CAD build for the part. Positions are in the model's coordinates, mm. A direction names the side the tool comes from. Give positions to 0.01 mm unless a question says otherwise; leave off trailing zeros. Write each loop counter-clockwise with the first axis right and the second up, starting at its lowest first coordinate (ties: lowest second). Pieces come first, ordered by that corner, then holes. Notation, with made-up numbers: (-10, -33.75) -> (-5, -33.75) arc R25 cw to (-5, -20.75) -> close; hole circle Ø9 at (-16, -36.5). An arc over 180 degrees is marked (long way). Answer as a JSON object with one key per item and string values.
```python
from build123d import *

# Parameters (mm, degrees)
ESQUISSE1_R        = 4.4
BOSS_EXTRU_1_DEPTH = 3
ESQUISSE2_R        = 7
BOSS_EXTRU_2_DEPTH = 2
ESQUISSE3_R        = 6.35
BOSS_EXTRU_3_DEPTH = 10
ESQUISSE4_R        = 4
BOSS_EXTRU_4_DEPTH = 7
ESQUISSE5_W        = 0.4
ESQUISSE5_H        = 2
BOSS_EXTRU_5_DEPTH = 5.8


with BuildPart() as part:
    # Esquisse1 → Boss.-Extru.1 (new body)
    with BuildSketch(Plane.XY):
        Circle(ESQUISSE1_R)
    extrude(amount=BOSS_EXTRU_1_DEPTH)

    # Esquisse2 → Boss.-Extru.2 (add)
    with BuildSketch(Plane.XY.offset(3)):
        Circle(ESQUISSE2_R)
    extrude(amount=BOSS_EXTRU_2_DEPTH)

    # Esquisse3 → Boss.-Extru.3 (add)
    with BuildSketch(Plane.XY.offset(5)):
        Circle(ESQUISSE3_R)
    extrude(amount=BOSS_EXTRU_3_DEPTH)

    # Esquisse4 → Boss.-Extru.4 (add)
    with BuildSketch(Plane.XY.offset(15)):
        Circle(ESQUISSE4_R)
    extrude(amount=BOSS_EXTRU_4_DEPTH)

    # Esquisse5 → Boss.-Extru.5 (add)
    with BuildSketch(Plane.XY.offset(22)):
        with Locations((-2.2, 0)):
            Rectangle(ESQUISSE5_W, ESQUISSE5_H)
        with Locations((2.2, 0)):
            Rectangle(ESQUISSE5_W, ESQUISSE5_H)
    extrude(amount=BOSS_EXTRU_5_DEPTH)


solid = part.part
```
1) 3-axis set-ups, long thin cutter, end or side, ignore diameter. For faces 1 (the cylindrical face through (-1.38, -6.2, 9.93)), 2 (the flat face through (0, -5, 3)), 3 (the flat face through (-2, 0, 25)): which of +Z, -Z, +X, -X, +Y, -Y reach the whole face in a straight line?
Model answer:
{"face 1": "+Z", "face 2": "-Z", "face 3": "+Z, +Y, -Y"}
2) Slice it at B-B (y = 0). List the corners of the cut face in (x, z).
Model answer:
{"outline": "(-7, 3) -> (-4.4, 3) -> (-4.4, 0) -> (4.4, 0) -> (4.4, 3) -> (7, 3) -> (7, 5) -> (6.35, 5) -> (6.35, 15) -> (4, 15) -> (4, 22) -> (2.4, 22) -> (2.4, 27.8) -> (2, 27.8) -> (2, 22) -> (-2, 22) -> (-2, 27.8) -> (-2.4, 27.8) -> (-2.4, 22) -> (-4, 22) -> (-4, 15) -> (-6.35, 15) -> (-6.35, 5) -> (-7, 5) -> close"}
3) Pin check, flat tips, straight feed: pin 1 (3 mm diameter, centred on x = -5.5, z = 12.5, fed in from -Y); pin 2 (5 mm diameter, centred on x = -3.5, z = 19, fed in from -Y); pin 3 (1.6 mm diameter, centred on y = -0.5, z = 24.5, fed in from +X). Stop position of each tip, or through.
Model answer:
{"pin 1": "stops at y = -4.93", "pin 2": "stops at y = -3.87", "pin 3": "stops at x = 2.4"}
4) Slice it at C-C (x = 0). List the corners of the cut face in (y, z), then the cut area to 3 significant figures.
Model answer:
{"outline": "(-7, 3) -> (-4.4, 3) -> (-4.4, 0) -> (4.4, 0) -> (4.4, 3) -> (7, 3) -> (7, 5) -> (6.35, 5) -> (6.35, 15) -> (4, 15) -> (4, 22) -> (-4, 22) -> (-4, 15) -> (-6.35, 15) -> (-6.35, 5) -> (-7, 5) -> close", "area": "237 mm2"}
5) Slice it at A-A (z = 23). List the corners of the cut face in (x, y), then the cut area to 3 significant figures.
Model answer:
{"outline": "(-2.4, -1) -> (-2, -1) -> (-2, 1) -> (-2.4, 1) -> close; (2, -1) -> (2.4, -1) -> (2.4, 1) -> (2, 1) -> close", "area": "1.60 mm2"}
6) Mould opens along X. For faces 4 (the flat face through (2, 0, 25)), 5 (the cylindrical face through (4.197, 1.322, 1.479)), 6 (the flat face through (3, -6, 5)), 7 (the flat face through (0, 0, 22)) say: released by +X, released by -X, zero draft, split by the parting line, or undercut.
Model answer:
{"face 4": "undercut", "face 5": "split by the parting line", "face 6": "zero draft", "face 7": "undercut"}
7) Slice it at D-D (z = 9.5). List the corners of the cut face in (x, y).
Model answer:
{"outline": "circle Ø12.7 at (0, 0)"}
8) Wall check: probe 1 along Z at (x, y) = (2.75, -0.75); probe 2 along Z at (x, y) = (3.5, 5.25); probe 3 along Y at (x, z) = (-0.25, 4.5). Give the ranges that are in metal, low to high.
Model answer:
{"probe 1": "z = 0 to 22", "probe 2": "z = 3 to 15", "probe 3": "y = -7 to 7"}
